```python
from build123d import *

# Parameters (mm, degrees)
SKETCH1_W           = 17.7
SKETCH1_H           = 15.16
SKETCH1_R           = 1.625
BOSS_EXTRUDE1_DEPTH = 0.75
SKETCH3_W           = 0.610582996
SKETCH3_H           = 3.110461755
SKETCH3_W_2         = 0.572421558
SKETCH3_W_3         = 0.542718384
SKETCH3_W_4         = 0.763228744
BOSS_EXTRUDE2_DEPTH = 0.2


with BuildPart() as part:
    # Sketch1 → Boss-Extrude1 (new, symmetric)
    with BuildSketch(Plane(origin=(0, 0, 0), x_dir=(1, 0, 0), z_dir=(0, 1, 0))):
        Rectangle(SKETCH1_W, SKETCH1_H)
        with Locations(Location((-6.52, -0.12, 0), (0, 0, 270))):
            Circle(SKETCH1_R, mode=Mode.SUBTRACT)
        with Locations(Location((6.52, -0.12, 0), (0, 0, 270))):
            Circle(SKETCH1_R, mode=Mode.SUBTRACT)
    extrude(amount=BOSS_EXTRUDE1_DEPTH, both=True)



with BuildPart() as body_2:
    # Sketch2 → Revolve1 (revolve)
    with BuildSketch(Plane(origin=(0, 0, 0), x_dir=(1, 0, 0), z_dir=(0, 1, 0)), mode=Mode.PRIVATE) as revolve1_sk:
        with BuildLine():
            Line((0, 9.28), (0, 18.13))
            ThreePointArc((0, 18.13), (-1.473784577, 17.707559711), (-2.499995, 16.568529884))
            Line((-2.499995, 16.568529884), (-2.499995, 9.914637604))
            Line((-2.499995, 9.914637604), (-2.862499587, 9.914637604))
            Line((-2.862499587, 9.914637604), (-2.862499587, 9.28))
            Line((-2.862499587, 9.28), (0, 9.28))
        make_face()
    revolve(revolve1_sk.sketch.rotate(Axis((0, 0, 0), (0, 0, -1)), 180), axis=Axis((0, 0, 0), (0, 0, -1)))


with BuildPart() as part_1:
    add(part.part)

    add(body_2.part)  # Boss-Extrude2 merges body 2
    # Sketch3 → Boss-Extrude2 (add)
    with BuildSketch(Plane(origin=(0, 0.75, 0), x_dir=(1, 0, 0), z_dir=(0, 1, 0))):
        with Locations((-1.975936472, 7.724769123)):
            Rectangle(SKETCH3_W, SKETCH3_H)
        with Locations((-0.945577667, 7.724769123)):
            Rectangle(SKETCH3_W_2, SKETCH3_H)
        with Locations((0.271359192, 7.724769123)):
            Rectangle(SKETCH3_W_3, SKETCH3_H)
        with Locations((1.6875615, 7.724769123)):
            Rectangle(SKETCH3_W_4, SKETCH3_H)
    extrude(amount=BOSS_EXTRUDE2_DEPTH)


solid = part_1.part
```
Geometry check sheet. Reference: the model listing, model coordinates, mm. A direction names the side the tool comes from. Coordinates: 2 decimals unless noted, no trailing zeros. Write each loop counter-clockwise with the first axis right and the second up, starting at its lowest first coordinate (ties: lowest second). Pieces come first, ordered by that corner, then holes. Notation, with made-up numbers: M -6,58 L 20,58 A19 ccw 20,81 Z; hole C 53.25,-35.5 d4. An arc over 180 degrees is marked long. Answer as a JSON object with one key per item and string values.
1. Section check A-A, the plane z = -9. Enter the section's corners in (x, y).
Answers below:
{"outline": "M -2.28,0.75 L -1.67,0.75 L -1.67,0.95 L -2.28,0.95 Z; M -1.23,0.75 L -0.66,0.75 L -0.66,0.95 L -1.23,0.95 Z; M 0,0.75 L 0.54,0.75 L 0.54,0.95 L 0,0.95 Z; M 1.31,0.75 L 2.07,0.75 L 2.07,0.95 L 1.31,0.95 Z"}
2. Section check B-B, the plane y = 0. Give the number of separate pieces and of enclosed holes in the cut face, plus the area to 3 significant figures.
Answers below:
{"separate pieces": "2", "enclosed holes": "2", "area": "294 mm²"}
3. Scan lines: L1, parallel to X at y = 0.4, z = 0.12 (3 decimals); L2, parallel to Z at x = 6.5, y = -0.3; L3, parallel to Y at x = -7, z = -5. Record each from-to range of solid material in increasing order.
Answers below:
{"L1": "x = -8.85 to -8.145, -4.895 to 4.895, 8.145 to 8.85", "L2": "z = -7.58 to -1.5, 1.74 to 7.58", "L3": "y = -0.75 to 0.75"}
4. Go/stop test with flat-tipped pins: pin 1 Ø3 at (x, z) = (-6.52, 0.12) entering from +Y; pin 2 Ø1.2 at (x, y) = (1, 0) entering from -Z. Record where each tip stops, or that it passes through.
Answers below:
{"pin 1": "passes through", "pin 2": "stops at z = -18.1"}
5. Section check C-C, the plane x = 6.52. Enter the section's corners in (y, z) (3 decimals).
Answers below:
{"outline": "M -0.75,-7.58 L 0.75,-7.58 L 0.75,-1.505 L -0.75,-1.505 Z; M -0.75,1.745 L 0.75,1.745 L 0.75,7.58 L -0.75,7.58 Z"}
6. Draft check along X on faces 1 (the cylindrical face through (-2.86, -0.13, -9.59)), 2 (the cylindrical face through (-8.106, -0.01, -0.232)), 3 (the flat face through (8.85, 0, 0)). Enter one of: released by +X, released by -X, zero draft, split by the parting line, or undercut.
Answers below:
{"face 1": "split by the parting line", "face 2": "undercut", "face 3": "released by +X"}
7. Tool access check on faces 4 (the flat face through (0, 0, -7.58)), 5 (the cylindrical face through (2.385, -0.751, -13.195)), 6 (the cylindrical face through (7.89, -0.01, 0.994)), 7 (the flat face through (0, -0.75, 0)). Record the directions out of +Z, -Z, +X, -X, +Y, -Y that give a thin tool (end or side, any length) a straight path to the whole face; none if there is none.
Answers below:
{"face 4": "+X, -X, -Y", "face 5": "-Z", "face 6": "+Y, -Y", "face 7": "+Z, +X, -X, -Y"}
8. Section check D-D, the plane z = 0.12. Enter the section's corners in (x, y) (3 decimals).
Answers below:
{"outline": "M -8.85,-0.75 L -8.145,-0.75 L -8.145,0.75 L -8.85,0.75 Z; M -4.895,-0.75 L 4.895,-0.75 L 4.895,0.75 L -4.895,0.75 Z; M 8.145,-0.75 L 8.85,-0.75 L 8.85,0.75 L 8.145,0.75 Z"}
